Could you check a few things on this model? Use its own coordinates, in mm. Round coordinates to 2 decimals unless told otherwise and drop trailing zeros. Loops run counter-clockwise (first coordinate to the right, second up) from the corner with the lowest first, then second, coordinate; pieces in that order, holes last. Notation, with made-up numbers: (21.5, 80) - (45.5, 80) arc R13 cw to (45.5, 95) - close; hole circle Ø5 at (-7, 85). An arc over 180 degrees is marked (long way). Answer as CSV lines item,"result". Start each with the question number.
1) I'm going to push a flat-ended pin straight in: pin 1 Ø4.5 at (x, y) = (44.9, -39.34) entering from -Z. Where does the tip first touch, or does it pass through?
2) Suppose I cut it at A-A, the plane y = -2.5. Write out the boundary of the cut face in (x, z).
3) We'd pull the mould along Y, two halves only. Please class faces 1 (the face through (0.962, -2.005, 0.805)), 2 (the face through (22, -41.91, 1)), 3 (the face through (43.15, -3.4, 0.8)), 4 (the face through (-2.54, -21, 1)): pulls with the +Y half, pulls with the -Y half, needs draft (parallel to the pull), parting line crosses it, or undercut.
4) Suppose I cut it at B-B, the plane x = 1. Write out the boundary of the cut face in (y, z), then the cut area to 3 significant figures.
5) Please list where these lines run through material, in increasing order: line 1 along X through (y, z) = (-39.5, 1.15); line 2 along X through (y, z) = (-40, 1); line 3 along Y through (x, z) = (44, 1.4).
6) Suppose I cut it at C-C, the plane z = 0.55. Write out the boundary of the cut face in (x, y), then the cut area to 3 significant figures.
Solid Edge part; units mm, degrees
sketch "Sketch1" plane through (0, 0, 0) normal (0, 0, 1) x (1, 0, 0)
  line L0 (-2.54, -0.91) -> (-2.54, -41.91)
  line L1 (-2.54, -41.91) -> (47.46, -41.91)
  line L2 (47.46, -41.91) -> (47.46, -0.91)
  line L3 (47.46, -0.91) -> (-2.54, -0.91)
extrude "Protrusion1" add sketch "Sketch1" along normal blind 1.5875
sketch "Sketch2" plane through (22.46, -21.41, 1.5875) normal (0, 0, 1) x (1, 0, 0)
  circle A0 centre (22.4383, 17.9298) radius 1.75
  circle A1 centre (22.4383, -17.9298) radius 1.75
  circle A2 centre (-22.4383, -17.9298) radius 1.75
  circle A3 centre (-22.4383, 17.9298) radius 1.75
extrude "ExtrudedCutout_1" cut sketch "Sketch2" against normal blind 33.274
Filled sheet:
1,pin 1,"z = 0"
2,outline,"(-2.54, 0) - (-1.43, 0) - (-1.43, 1.59) - (-2.54, 1.59) - close; (1.47, 0) - (43.45, 0) - (43.45, 1.59) - (1.47, 1.59) - close; (46.35, 0) - (47.46, 0) - (47.46, 1.59) - (46.35, 1.59) - close"
3,face 1,"undercut"
3,face 2,"pulls with the -Y half"
3,face 3,"undercut"
3,face 4,"needs draft"
4,outline,"(-41.91, 0) - (-40.79, 0) - (-40.79, 1.59) - (-41.91, 1.59) - close; (-37.89, 0) - (-4.93, 0) - (-4.93, 1.59) - (-37.89, 1.59) - close; (-2.03, 0) - (-0.91, 0) - (-0.91, 1.59) - (-2.03, 1.59) - close"
4,area,"55.9 mm²"
5,line 1,"-2.54 to -1.72, 1.76 to 43.16, 46.64 to 47.46"
5,line 2,"-2.54 to -1.6, 1.64 to 43.28, 46.52 to 47.46"
5,line 3,"-41.91 to -40.84, -37.84 to -4.98, -1.98 to -0.91"
6,outline,"(-2.54, -41.91) - (47.46, -41.91) - (47.46, -0.91) - (-2.54, -0.91) - close; hole circle Ø3.5 at (0.02, -39.34); hole circle Ø3.5 at (0.02, -3.48); hole circle Ø3.5 at (44.9, -39.34); hole circle Ø3.5 at (44.9, -3.48)"
6,area,"2,010 mm²"
